Geometry check sheet. Reference: drawing and pictorial views, mm from the part's lowest x, y, z. A direction names the side the tool comes from. Round coordinates to 2 decimals unless told otherwise and drop trailing zeros. Write each loop counter-clockwise with the first axis right and the second up, starting at its lowest first coordinate (ties: lowest second). Pieces come first, ordered by that corner, then holes. Notation, with made-up numbers: M 39,-23.5 L 88,-23.5 A25 cw 88,11.5 Z; hole C 12.5,64.25 d2. An arc over 180 degrees is marked long. One line per question, with ' | ' between items.
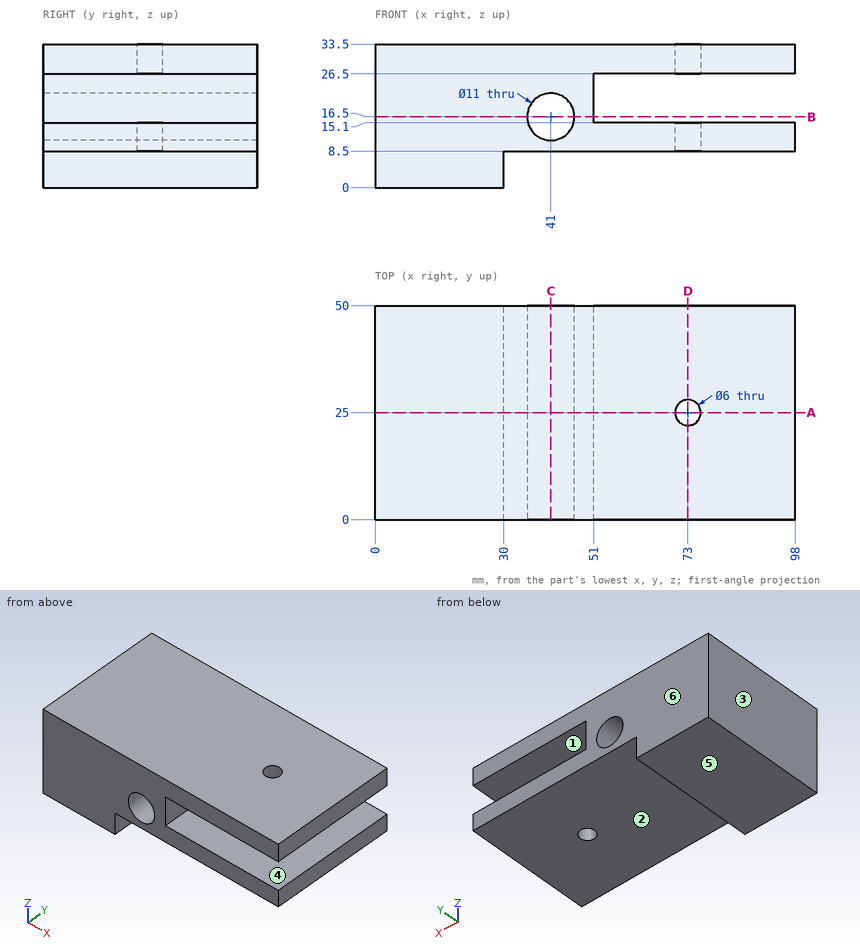
1. Tool access check on the marked faces 1, 2 and 3. Record the directions out of +Z, -Z, +X, -X, +Y, -Y that give a thin tool (end or side, any length) a straight path to the whole face; none if there is none.
Results:
face 1: +X, +Y, -Y | face 2: -Z, +X, +Y, -Y | face 3: +Z, -Z, -X, +Y, -Y
2. Section check A-A, the plane y = 25. Record the cut outline in (x, z).
Results:
outline: M 0,0 L 30,0 L 30,8.5 L 70,8.5 L 70,15.1 L 51,15.1 L 51,26.5 L 70,26.5 L 70,33.5 L 0,33.5 Z; M 76,8.5 L 98,8.5 L 98,15.1 L 76,15.1 Z; M 76,26.5 L 98,26.5 L 98,33.5 L 76,33.5 Z; hole C 41,16.5 d11
3. Mould release check, pull along Z, two halves, no side actions. Record for the marked faces 4, 5 and 6: pulls with the +Z half, pulls with the -Z half, needs draft (parallel to the pull), parting line crosses it, or undercut.
Results:
face 4: undercut | face 5: pulls with the -Z half | face 6: needs draft
4. Section check B-B, the plane z = 16.5. Record the cut outline in (x, y), then the cut area to 3 significant figures.
Results:
outline: M 0,0 L 35.5,0 L 35.5,50 L 0,50 Z; M 46.5,0 L 51,0 L 51,50 L 46.5,50 Z | area: 2,000 mm2
5. Go/stop test with flat-tipped pins: P1, Ø5, axis at x = 73, y = 25, coming from the +Z side; P2, Ø7, axis at y = 19.5, z = 4, coming from the +X side; P3, Ø5.5, axis at y = 31.5, z = 21, coming from the +X side; P4, Ø12, axis at x = 67, y = 36, coming from the -Z side. Record where each tip stops, or that it passes through.
Results:
P1: passes through | P2: stops at x = 30 | P3: stops at x = 51 | P4: stops at z = 8.5
6. Section check C-C, the plane x = 41. Record the cut outline in (y, z), then the cut area to 3 significant figures.
Results:
outline: M 0,8.5 L 50,8.5 L 50,11 L 0,11 Z; M 0,22 L 50,22 L 50,33.5 L 0,33.5 Z | area: 700 mm2
7. Section check D-D, the plane x = 73. Record the cut outline in (y, z).
Results:
outline: M 0,8.5 L 22,8.5 L 22,15.1 L 0,15.1 Z; M 0,26.5 L 22,26.5 L 22,33.5 L 0,33.5 Z; M 28,8.5 L 50,8.5 L 50,15.1 L 28,15.1 Z; M 28,26.5 L 50,26.5 L 50,33.5 L 28,33.5 Z
8. Thickness scan on line 1 (Z direction, x = 41, y = 29.5); line 2 (Z direction, x = 78.5, y = 8.5); line 3 (Y direction, x = 73, z = 31). Record the ranges inside material, lowest first.
Results:
line 1: z = 8.5 to 11, 22 to 33.5 | line 2: z = 8.5 to 15.1, 26.5 to 33.5 | line 3: y = 0 to 22, 28 to 50
